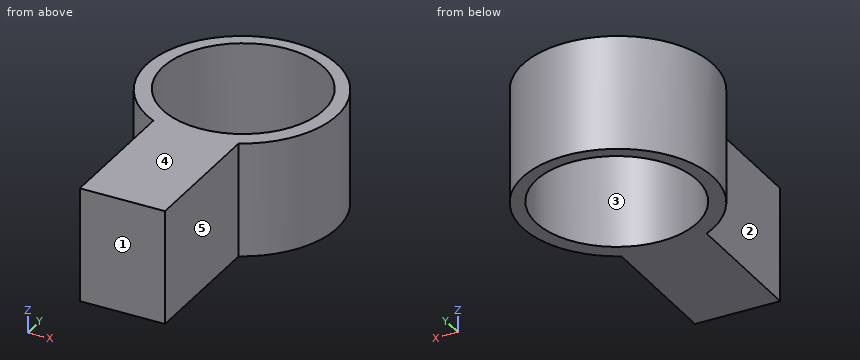
from build123d import *

# Parameters (mm, degrees)
RESSALTO_EXTRUS_O1_DEPTH = 18
ESBO_O3_R                = 12.668025565
CORTE_EXTRUS_O2_DEPTH    = 58.275422957


with BuildPart() as part:
    # Esboço1 → Ressalto-extrusão1 (new body)
    with BuildSketch(Plane.XY):
        with BuildLine():
            Line((0, 0), (0, 21.43532158))
            ThreePointArc((0, 21.43532158), (6.703057614, 49.854301371), (13.406115228, 21.43532158))
            Line((13.406115228, 21.43532158), (13.406115228, 0))
            Line((13.406115228, 0), (0, 0))
        make_face()
    extrude(amount=RESSALTO_EXTRUS_O1_DEPTH)

    # Esboço3 → Corte-extrusão2 (cut, through all)
    with BuildSketch(Plane.XY.offset(18)):
        with Locations((6.703057614, 35.210084405)):
            Circle(ESBO_O3_R)
    extrude(amount=-CORTE_EXTRUS_O2_DEPTH, mode=Mode.SUBTRACT)


solid = part.part
Input: part model. Units: mm. Frame: model coordinates. Face numbers are marked on the shaded views. A direction names the side the tool comes from. Coordinates: 2 decimals unless noted, no trailing zeros. Write each loop counter-clockwise with the first axis right and the second up, starting at its lowest first coordinate (ties: lowest second). Pieces come first, ordered by that corner, then holes. Notation, with made-up numbers: M 1,-28 L 19,-28 A16 ccw 19,-23 Z; hole C 37.5,7.25 d2. An arc over 180 degrees is marked long. Answer as a JSON object with one key per item and string values. Group by question number.
(1) Contact query for flat-ended pins moving along their axis: P1, Ø8, axis at x = -5, z = 2.5, coming from the -Y side; P2, Ø6, axis at y = 9.5, z = 11.5, coming from the +X side; P3, Ø2, axis at y = 14.5, z = 3.5, coming from the -X side; P4, Ø12, axis at x = 2.5, y = 33.5, coming from the -Z side. Output: stop coordinate, or through.
(2) Section D-D on y = 17.5. Output: boundary loops of the cut face in (x, z), plus the area to 3 significant figures.
(3) Section B-B on x = 16. Output: boundary loops of the cut face in (y, z).
(4) Section A-A on y = 33. Output: boundary loops of the cut face in (x, z).
(5) Section C-C on z = 6.5. Output: boundary loops of the cut face in (x, y).
(6) Mould query, pull axis Y, two halves, no side actions, for the marked faces 1, 2 and 3. Classes: pulls with the +Y half, pulls with the -Y half, needs draft (parallel to the pull), parting line crosses it, or undercut.
(7) Ray query, line 1 along Y through (x, z) = (7, 3.5); line 2 along X through (y, z) = (5, 14.25); line 3 along Y through (x, z) = (1.5, 12.25). Return the intervals inside material, ascending. Write a range as [from, to].
(8) Set-up query: the marked faces 4 and 5. Return all of +Z, -Z, +X, -X, +Y, -Y with unobstructed straight access to the full face (end or side cutting, diameter ignored); none if empty.
Result set:
{
 "1": {"P1": "stops at y = 21.98", "P2": "stops at x = 13.41", "P3": "stops at x = 0", "P4": "passes through"},
 "2": {"outline": "M 0,0 L 13.41,0 L 13.41,18 L 0,18 Z", "area": "241 mm2"},
 "3": {"outline": "M 23.08,0 L 26.61,0 L 26.61,18 L 23.08,18 Z; M 43.82,0 L 46.63,0 L 46.63,18 L 43.82,18 Z"},
 "4": {"outline": "M -8.18,0 L -5.77,0 L -5.77,18 L -8.18,18 Z; M 19.18,0 L 21.59,0 L 21.59,18 L 19.18,18 Z"},
 "5": {"outline": "M 0,0 L 13.41,0 L 13.41,21.44 A15 ccw long 0,21.44 Z; hole C 6.7,35.21 d25.34"},
 "6": {"face 1": "pulls with the -Y half", "face 2": "needs draft", "face 3": "undercut"},
 "7": {"line 1": "y = [0, 22.55], [47.87, 49.85]", "line 2": "x = [0, 13.41]", "line 3": "y = [0, 23.66], [46.76, 48.92]"},
 "8": {"face 4": "+Z, +X, -X, +Y, -Y", "face 5": "+Z, -Z, +X, -Y"}
}
